from build123d import *

# Parameters (mm, degrees)
SKETCH1_R           = 17.5
BOSS_EXTRUDE1_DEPTH = 1.5
BOSS_EXTRUDE2_START = -1.5
SKETCH2_R           = 16
BOSS_EXTRUDE2_DEPTH = 5
SKETCH3_R           = 12
BOSS_EXTRUDE3_DEPTH = 6
SKETCH4_R           = 7
CUT_EXTRUDE1_DEPTH  = 28.726341266
SKETCH5_R           = 1.5
CUT_EXTRUDE2_DEPTH  = 26.588083164
CHAMFER1_SIZE       = 0.75
FILLET1_R           = 0.5
SKETCH6_R           = 1.5
CUT_EXTRUDE3_DEPTH  = 26.860201082
CIRPATTERN1_COUNT   = 4


with BuildPart() as part:
    # Sketch1 → Boss-Extrude1 (new body)
    with BuildSketch(Plane.XY):
        Circle(SKETCH1_R)
    extrude(amount=BOSS_EXTRUDE1_DEPTH)

    # Sketch2 → Boss-Extrude2 (add)
    with BuildSketch(Plane.XY.offset(1.5).offset(BOSS_EXTRUDE2_START)):
        Circle(SKETCH2_R)
    extrude(amount=-BOSS_EXTRUDE2_DEPTH)

    # Sketch3 → Boss-Extrude3 (add)
    with BuildSketch(Plane.XY.offset(1.5)):
        with Locations((0, -3.5)):
            Circle(SKETCH3_R)
    extrude(amount=BOSS_EXTRUDE3_DEPTH)

    # Sketch4 → Cut-Extrude1 (cut, through all)
    with BuildSketch(Plane.XY.offset(7.5)):
        with Locations((0, -3.5)):
            Circle(SKETCH4_R)
    extrude(amount=-CUT_EXTRUDE1_DEPTH, mode=Mode.SUBTRACT)

    # Sketch5 → Cut-Extrude2 (cut, through all)
    with BuildSketch(Plane.XY.offset(1.5)):
        with Locations((-8, 9.5)):
            Circle(SKETCH5_R)
        with Locations((8, 9.5)):
            Circle(SKETCH5_R)
    extrude(amount=-CUT_EXTRUDE2_DEPTH, mode=Mode.SUBTRACT)

    # Chamfer1
    chamfer1_edges = [part.edges().sort_by_distance(p)[0] for p in [
        (-9.5, 9.5, 1.5),
        (6.5, 9.5, 1.5),
    ]]
    chamfer(chamfer1_edges, length=CHAMFER1_SIZE)

    # Fillet1
    fillet1_edges = [part.edges().sort_by_distance(p)[0] for p in [
        (-12, -3.5, 1.5),
        (-12, -3.5, 7.5),
    ]]
    fillet(fillet1_edges, radius=FILLET1_R)

    # Sketch6 → Cut-Extrude3 (cut, symmetric)
    with BuildSketch(Plane(origin=(0, 0, 0), x_dir=(0, 0, -1), z_dir=(1, 0, 0))):
        with Locations((-4.5, -3.5)):
            Circle(SKETCH6_R)
    cut_extrude3 = extrude(amount=CUT_EXTRUDE3_DEPTH, both=True, mode=Mode.SUBTRACT)

    # CirPattern1: Cut-Extrude3 ×4 about axis
    cirpattern1_axis = Axis((0, -3.5, 7.5), (0, 0, -1))
    for i in range(1, CIRPATTERN1_COUNT):
        add(cut_extrude3.rotate(cirpattern1_axis, i * 360 / CIRPATTERN1_COUNT), mode=Mode.SUBTRACT)


solid = part.part
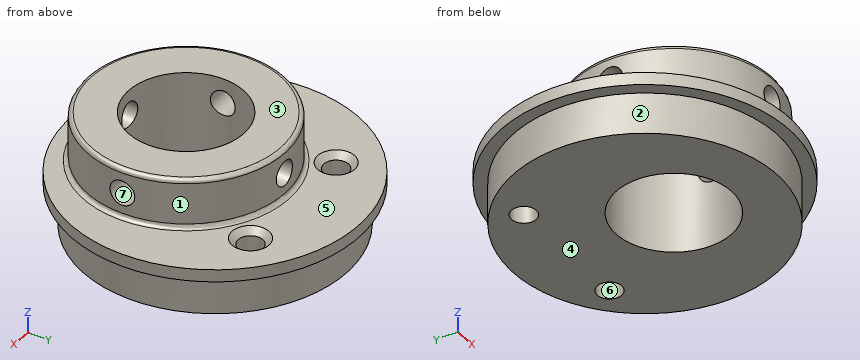
CAD build for the part. Positions are in the model's coordinates, mm. Face numbers are marked on the shaded views. A direction names the side the tool comes from. Round coordinates to 2 decimals unless told otherwise and drop trailing zeros. Write each loop counter-clockwise with the first axis right and the second up, starting at its lowest first coordinate (ties: lowest second). Pieces come first, ordered by that corner, then holes.
(1) Drop flat-ended pins along their axis: P1, Ø3.5, axis at y = -3.5, z = 4.5, coming from the +X side; P2, Ø1, axis at y = -3, z = 0.5, coming from the -X side; P3, Ø1, axis at x = 9.5, z = -1.5, coming from the +Y side. Give the stop position or say it passes through.
(2) Slice it at B-B, the plane z = 4.5. Write the cut outline in (x, y).
(3) Slice it at A-A, the plane y = 9.5. Write the cut outline in (x, z), and give its area (3 significant figures).
(4) Probe line 1 along Y through (x, z) = (8.9, 4.5); line 2 along Z through (x, y) = (-6.5, 6.5); line 3 along X through (y, z) = (-0.5, 6.25). List the from-to ranges inside material, lowest first.
(5) Mould opens along Z. For the marked faces 4, 5, 6 and 7 say: pulls with the +Z half, pulls with the -Z half, needs draft (parallel to the pull), parting line crosses it, or undercut.
(6) Slice it at C-C, the plane x = 8. Count the separate pieces of the cut face and the enclosed holes in it, and give its area (3 significant figures).
(7) Slice it at D-D, the plane z = -0.5. Write the cut outline in (x, y).
(8) 3-axis set-ups, long thin cutter, end or side, ignore diameter. For the marked faces 1, 2 and 3: which of +Z, -Z, +X, -X, +Y, -Y reach the whole face in a straight line?
From the geometry:
1. P1: stops at x = 12
1. P2: stops at x = -17.32
1. P3: stops at y = 13.23
2. outline: (-11.91, -5) arc R12 ccw to (-1.5, -15.41) - (-1.5, -10.34) arc R7 cw to (-6.84, -5) - close; (-11.91, -2) - (-6.84, -2) arc R7 cw to (-1.5, 3.34) - (-1.5, 8.41) arc R12 ccw to start; (1.5, -15.41) arc R12 ccw to (11.91, -5) - (6.84, -5) arc R7 cw to (1.5, -10.34) - close; (1.5, 3.34) arc R7 cw to (6.84, -2) - (11.91, -2) arc R12 ccw to (1.5, 8.41) - close
3. outline: (-14.7, 0) - (-12.87, 0) - (-12.87, -5) - (-9.5, -5) - (-9.5, 0.75) - (-10.25, 1.5) - (-14.7, 1.5) - close; (-6.5, -5) - (6.5, -5) - (6.5, 0.75) - (5.75, 1.5) - (-5.75, 1.5) - (-6.5, 0.75) - close; (9.5, -5) - (12.87, -5) - (12.87, 0) - (14.7, 0) - (14.7, 1.5) - (10.25, 1.5) - (9.5, 0.75) - close
3. area: 133 mm2
4. line 1: y = -11.55 to -5, -2 to 4.55
4. line 2: z = -5 to 7.26
4. line 3: x = -11.62 to -6.32, 6.32 to 11.62
5. face 4: pulls with the -Z half
5. face 5: pulls with the +Z half
5. face 6: needs draft
5. face 7: undercut
6. separate pieces: 2
6. enclosed holes: 1
6. area: 265 mm2
7. outline: circle Ø32 at (0, 0); hole circle Ø3 at (-8, 9.5); hole circle Ø14 at (0, -3.5); hole circle Ø3 at (8, 9.5)
8. face 1: +Z
8. face 2: -Z
8. face 3: +Z, +X, -X, +Y, -Y
